Check sheet for the modelled part. Datum: model origin and axes. Units: mm. A direction names the side the tool comes from. Round coordinates to 2 decimals unless told otherwise and drop trailing zeros. Write each loop counter-clockwise with the first axis right and the second up, starting at its lowest first coordinate (ties: lowest second). Pieces come first, ordered by that corner, then holes. Notation, with made-up numbers: M -0.5,1 L 57.5,1 A32 cw 57.5,34 Z; hole C 27.25,56 d1. An arc over 180 degrees is marked long. One line per item, written item: value.
from build123d import *

# Parameters (mm, degrees)
SKETCH1_W                       = 88.9
SKETCH1_H                       = 76.2
BOSS_EXTRUDE1_DEPTH             = 37.592
CUT_EXTRUDE1_REACH              = 124.975
SHELL1_T                        = -3.175
SKETCH16_W                      = 12.664560545
SKETCH16_H                      = 36.83
SKETCH16_W_2                    = 12.692903968
BOSS_EXTRUDE4_DEPTH             = 63.5
BOSS_EXTRUDE4_DIRECTION_2_REACH = 124.975
CUT_EXTRUDE2_REACH              = 171.328
SKETCH18_R                      = 14.605
CUT_EXTRUDE3_REACH              = 171.339
SKETCH20_R                      = 13.97
SKETCH20_R_2                    = 1.905
CUT_EXTRUDE4_DEPTH              = 175.485983575
FILLET2_R                       = 6.35


with BuildPart() as part:
    # Sketch1 → Boss-Extrude1 (new body)
    with BuildSketch(Plane(origin=(0, 0, 0), x_dir=(1, 0, 0), z_dir=(0, 1, 0))):
        with Locations((-44.45, 38.1)):
            Rectangle(SKETCH1_W, SKETCH1_H)
    extrude(amount=-BOSS_EXTRUDE1_DEPTH)

    # Sketch2 → Cut-Extrude1 (cut, up to next)
    with BuildSketch(Plane.XY, mode=Mode.PRIVATE) as cut_extrude1_sk1:
        with BuildLine():
            ThreePointArc((-49.926198023, -37.592), (-71.560931997, -32.647565517), (-88.9, -18.796))
            Line((-88.9, -18.796), (-88.9, -37.592))
            Line((-88.9, -37.592), (-49.926198023, -37.592))
        make_face()
    cut_extrude1_tool1 = extrude(cut_extrude1_sk1.sketch, amount=-CUT_EXTRUDE1_REACH, mode=Mode.PRIVATE) & part.part
    # Sketch2 → Cut-Extrude1 (cut, up to next)
    with BuildSketch(Plane.XY, mode=Mode.PRIVATE) as cut_extrude1_sk2:
        with BuildLine():
            Line((0, -37.592), (0, 0))
            Line((0, 0), (-5.972186469, -11.208166165))
            ThreePointArc((-5.972186469, -11.208166165), (-24.293885313, -30.489622768), (-49.926198023, -37.592))
            Line((-49.926198023, -37.592), (0, -37.592))
        make_face()
    cut_extrude1_tool2 = extrude(cut_extrude1_sk2.sketch, amount=-CUT_EXTRUDE1_REACH, mode=Mode.PRIVATE) & part.part
    add(cut_extrude1_tool1.solids().sort_by_distance((-79.562366, -32.198077, 0))[0], mode=Mode.SUBTRACT)
    add(cut_extrude1_tool2.solids().sort_by_distance((-11.384711, -27.029682, 0))[0], mode=Mode.SUBTRACT)

    # Shell1
    shell1_openings = [part.faces().sort_by_distance(p)[0] for p in [
        (-44.45, 0, -38.1),
    ]]
    offset(amount=SHELL1_T, openings=shell1_openings, kind=Kind.INTERSECTION)

    # Sketch16 → Boss-Extrude4 (add)
    with BuildSketch(Plane.ZY.offset(88.9)):
        with Locations((-6.332280273, -18.415)):
            Rectangle(SKETCH16_W, SKETCH16_H)
        with Locations((-69.853548016, -18.415)):
            Rectangle(SKETCH16_W_2, SKETCH16_H)
    extrude(amount=BOSS_EXTRUDE4_DEPTH)

    # Sketch16 → Boss-Extrude4 direction 2 (add, up to next)
    with BuildSketch(Plane.ZY.offset(88.9), mode=Mode.PRIVATE) as boss_extrude4_direction_2_sk1:
        with Locations((-6.332280273, -18.415)):
            Rectangle(SKETCH16_W, SKETCH16_H)
    boss_extrude4_direction_2_tool1 = extrude(boss_extrude4_direction_2_sk1.sketch, amount=-BOSS_EXTRUDE4_DIRECTION_2_REACH, mode=Mode.PRIVATE) - part.part
    # Sketch16 → Boss-Extrude4 direction 2 (add, up to next)
    with BuildSketch(Plane.ZY.offset(88.9), mode=Mode.PRIVATE) as boss_extrude4_direction_2_sk2:
        with Locations((-69.853548016, -18.415)):
            Rectangle(SKETCH16_W_2, SKETCH16_H)
    boss_extrude4_direction_2_tool2 = extrude(boss_extrude4_direction_2_sk2.sketch, amount=-BOSS_EXTRUDE4_DIRECTION_2_REACH, mode=Mode.PRIVATE) - part.part
    add(boss_extrude4_direction_2_tool1.solids().sort_by_distance((-88.9, -18.415, -6.33228))[0])
    add(boss_extrude4_direction_2_tool2.solids().sort_by_distance((-88.9, -18.415, -69.853548))[0])

    # Sketch18 → Cut-Extrude2 (cut, up to next)
    with BuildSketch(Plane.XY.offset(-63.507096032), mode=Mode.PRIVATE) as cut_extrude2_sk1:
        with Locations((-123.825, -18.415)):
            Circle(SKETCH18_R)
    cut_extrude2_tool1 = extrude(cut_extrude2_sk1.sketch, amount=-CUT_EXTRUDE2_REACH, mode=Mode.PRIVATE) & part.part
    add(cut_extrude2_tool1.solids().sort_by_distance((-123.825, -18.415, -63.507096))[0], mode=Mode.SUBTRACT)

    # Sketch20 → Cut-Extrude3 (cut, up to next)
    with BuildSketch(Plane(origin=(0, 0, -12.664560545), x_dir=(-1, 0, 0), z_dir=(0, 0, -1)), mode=Mode.PRIVATE) as cut_extrude3_sk1:
        with Locations((123.825, -18.415)):
            Circle(SKETCH20_R)
    cut_extrude3_tool1 = extrude(cut_extrude3_sk1.sketch, amount=-CUT_EXTRUDE3_REACH, mode=Mode.PRIVATE) & part.part
    # Sketch20 → Cut-Extrude3 (cut, up to next)
    with BuildSketch(Plane(origin=(0, 0, -12.664560545), x_dir=(-1, 0, 0), z_dir=(0, 0, -1)), mode=Mode.PRIVATE) as cut_extrude3_sk2:
        with Locations((137.295382, -4.944618)):
            Circle(SKETCH20_R_2)
    cut_extrude3_tool2 = extrude(cut_extrude3_sk2.sketch, amount=-CUT_EXTRUDE3_REACH, mode=Mode.PRIVATE) & part.part
    # Sketch20 → Cut-Extrude3 (cut, up to next)
    with BuildSketch(Plane(origin=(0, 0, -12.664560545), x_dir=(-1, 0, 0), z_dir=(0, 0, -1)), mode=Mode.PRIVATE) as cut_extrude3_sk3:
        with Locations((137.295382, -31.885382)):
            Circle(SKETCH20_R_2)
    cut_extrude3_tool3 = extrude(cut_extrude3_sk3.sketch, amount=-CUT_EXTRUDE3_REACH, mode=Mode.PRIVATE) & part.part
    # Sketch20 → Cut-Extrude3 (cut, up to next)
    with BuildSketch(Plane(origin=(0, 0, -12.664560545), x_dir=(-1, 0, 0), z_dir=(0, 0, -1)), mode=Mode.PRIVATE) as cut_extrude3_sk4:
        with Locations((110.354618, -31.885382)):
            Circle(SKETCH20_R_2)
    cut_extrude3_tool4 = extrude(cut_extrude3_sk4.sketch, amount=-CUT_EXTRUDE3_REACH, mode=Mode.PRIVATE) & part.part
    # Sketch20 → Cut-Extrude3 (cut, up to next)
    with BuildSketch(Plane(origin=(0, 0, -12.664560545), x_dir=(-1, 0, 0), z_dir=(0, 0, -1)), mode=Mode.PRIVATE) as cut_extrude3_sk5:
        with Locations((110.354618, -4.944618)):
            Circle(SKETCH20_R_2)
    cut_extrude3_tool5 = extrude(cut_extrude3_sk5.sketch, amount=-CUT_EXTRUDE3_REACH, mode=Mode.PRIVATE) & part.part
    add(cut_extrude3_tool1.solids().sort_by_distance((-123.825, -18.415, -12.664561))[0], mode=Mode.SUBTRACT)
    add(cut_extrude3_tool2.solids().sort_by_distance((-137.295382, -4.944618, -12.664561))[0], mode=Mode.SUBTRACT)
    add(cut_extrude3_tool3.solids().sort_by_distance((-137.295382, -31.885382, -12.664561))[0], mode=Mode.SUBTRACT)
    add(cut_extrude3_tool4.solids().sort_by_distance((-110.354618, -31.885382, -12.664561))[0], mode=Mode.SUBTRACT)
    add(cut_extrude3_tool5.solids().sort_by_distance((-110.354618, -4.944618, -12.664561))[0], mode=Mode.SUBTRACT)

    # Sketch22 → Cut-Extrude4 (cut, through all)
    with BuildSketch(Plane(origin=(0, 0, -76.2), x_dir=(-1, 0, 0), z_dir=(0, 0, -1))):
        with BuildLine():
            Line((139.329278278, 0), (152.4, 0))
            Line((152.4, 0), (152.4, -36.83))
            Line((152.4, -36.83), (139.329278278, -36.83))
            ThreePointArc((139.329278278, -36.83), (146.957021029, -18.415), (139.329278278, 0))
        make_face()
    extrude(amount=-CUT_EXTRUDE4_DEPTH, mode=Mode.SUBTRACT)

    # Fillet2
    fillet2_edges = [part.edges().sort_by_distance(p)[0] for p in [
        (-75.401646537, -30.583390997, -63.507096032),
        (-75.401646537, -30.583390997, -12.664560545),
        (-88.9, -9.398, -63.507096032),
        (-88.9, -9.398, -12.664560545),
        (-6.185914068, -4.857559774, -73.025),
        (-6.185914068, -4.857559774, -3.175),
        (-85.725, -8.83323263, -73.025),
        (-45.133487238, -34.170041352, -73.025),
        (-85.725, -17.66646526, -38.1),
        (-85.725, -8.83323263, -3.175),
        (-45.133487238, -34.170041352, -3.175),
    ]]
    fillet(fillet2_edges, radius=FILLET2_R - 0.0001)  # a hair under: the kernel refuses the full size


solid = part.part
Q1. Access from +Z, -Z, +X, -X, +Y, -Y to the whole of each face (thin tool, end or side, straight path). Record for faces 4 (the flat face through (-46, -11, -3.175)), 5 (the cylindrical face through (-109.894, -14.028, -69.765)), 6 (the flat face through (-100, -36.83, -69)), 7 (the flat face through (-88.9, -9, -38)), 8 (the cylindrical face through (-111.38, -30.28, -6.42)).
Completed:
face 4: +Y
face 5: -Z
face 6: +Z, -Z, -X, -Y
face 7: -X, +Y, -Y
face 8: +Z
Q2. Draft check along X on faces 1 (the cylindrical face through (-7.907, -4.028, -71.214)), 2 (the cylindrical face through (-90.809, -10.323, -61.696)), 3 (the flat face through (-2.944, -5.526, -37.567)). Enter one of: pulls with the +X half, pulls with the -X half, needs draft (parallel to the pull), parting line crosses it, or undercut.
Completed:
face 1: undercut
face 2: pulls with the -X half
face 3: pulls with the +X half
Q3. Sectioned sample at D-D on z = -59. Enter the section's corners in (x, y) (1 decimal).
Completed:
outline: M -89.2,-18.9 A50.1 ccw -60.1,-36.8 L -58.6,-36.8 A49.8 ccw -6,-11.2 L 0,0 L -3.6,0 L -8.8,-9.7 A46.6 cw -84,-19.6 A6.3 cw -85.7,-15.3 L -85.7,0 L -89.2,0 Z
Q4. Depth check by flat-ended pin: P1, Ø9.5, axis at x = -96, z = -68, coming from the -Y side; P2, Ø1.5, axis at x = -43, z = -37, coming from the +Y side; P3, Ø5, axis at x = -60, z = -60.5, coming from the -Y side. Enter the tip coordinate at first touch or a pass-through.
Completed:
P1: y = -36.83
P2: y = -33.78
P3: y = -37.01
Q5. Sectioned sample at C-C on z = -6.5. Enter the section's corners in (x, y) (1 decimal).
Completed:
outline: M -139.3,-36.8 L -58.6,-36.8 A49.8 ccw -6,-11.2 L 0,0 L -4.5,0 L -9.5,-9.4 A45.9 cw -83.5,-19.1 A5.6 cw -85,-15.3 L -85,0 L -139.3,0 A26 ccw Z; hole C -137.3,-31.9 d3.8; hole C -137.3,-4.9 d3.8; hole C -123.8,-18.4 d27.9; hole C -110.4,-31.9 d3.8; hole C -110.4,-4.9 d3.8
Q6. Sectioned sample at A-A on z = -24. Enter the section's corners in (x, y) (1 decimal), and give its area (3 significant figures).
Completed:
outline: M -88.9,-18.8 A49.8 ccw -6,-11.2 L 0,0 L -3.6,0 L -8.8,-9.7 A46.6 cw -84,-19.6 A6.3 cw -85.7,-15.3 L -85.7,0 L -88.9,0 Z
area: 398 mm^2
Q7. Scan lines: line 1 (Z direction, x = -69, y = -10.5) (3 decimals); line 2 (Z direction, x = -97.5, y = -35); line 3 (Y direction, x = -119.5, z = -73). Record each from-to range of solid material in increasing order. Write a range as [from, to].
Completed:
line 1: [-76.2, -73.025], [-3.175, 0]
line 2: [-76.2, -63.51], [-12.66, 0]
line 3: [-36.83, -32.36], [-4.47, 0]
Q8. Sectioned sample at B-B on y = -26. State how many separate pieces and enclosed holes the cut face has, and give its area (3 significant figures).
Completed:
separate pieces: 3
enclosed holes: 1
area: 2,230 mm^2
